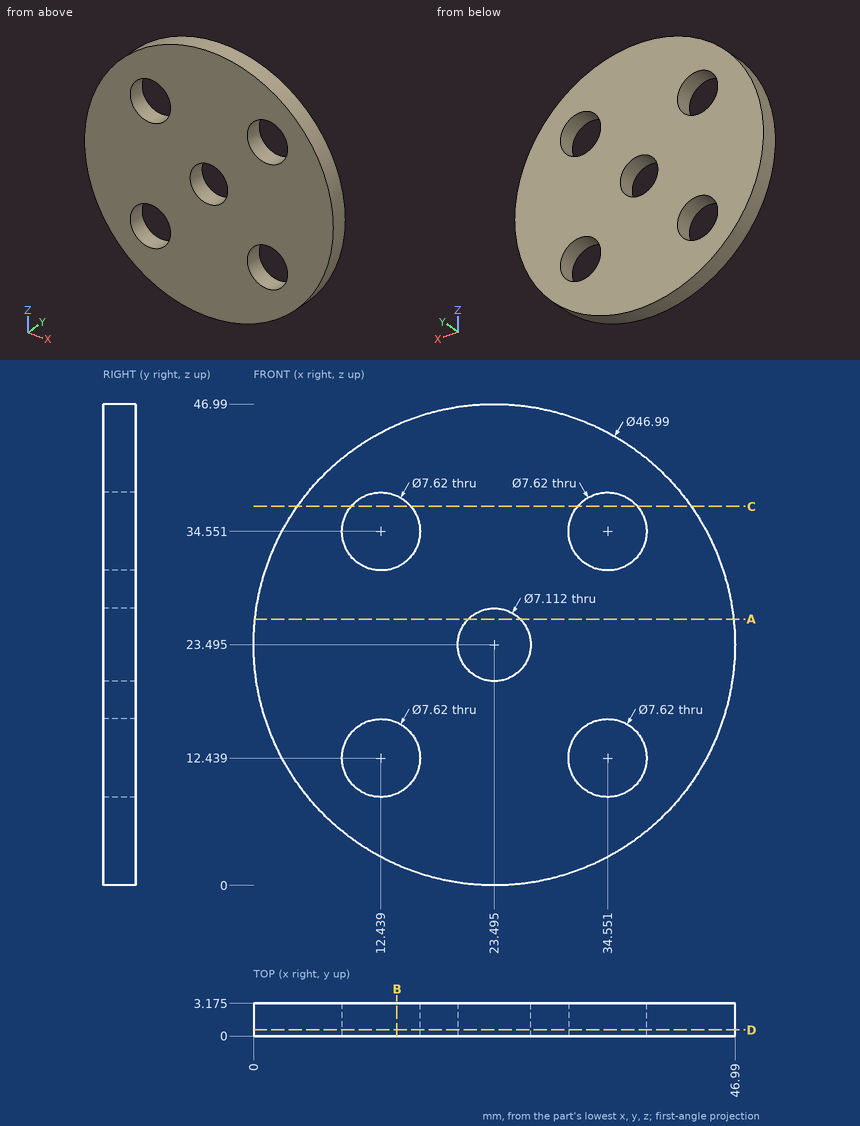
Study the drawing (mm; zero at the part's minimum x, y, z) and answer. Coordinates: 2 decimals unless noted, no trailing zeros. Write each loop counter-clockwise with the first axis right and the second up, starting at its lowest first coordinate (ties: lowest second). Pieces come first, ordered by that corner, then holes. Notation, with made-up numbers: (41.5, 45.5) - (71.5, 45.5) arc R17 cw to (71.5, 62.5) - close; hole circle Ø6 at (6, -38). An arc over 180 degrees is marked (long way). Return JSON: item names as keys, results as strings. Group by question number.
1. A cutting plane is placed at B-B, the plane x = 14. Determine the outline of the cut face in (y, z) (1 decimal), plus the area to 3 significant figures.
2. A cutting plane is placed at A-A, the plane z = 26. Determine the outline of the cut face in (x, y) (3 decimals), plus the area to 3 significant figures.
3. A cutting plane is placed at C-C, the plane z = 37. Determine the outline of the cut face in (x, y) (1 decimal).
4. Straight lines are drawn through the part: L1, parallel to X at y = 0.5, z = 10; L2, parallel to Z at x = 38, y = 2.4; L3, parallel to Z at x = 37, y = 1.55. For each, find the intervals that lie inside material, in ascending order.
5. A cutting plane is placed at D-D, the plane y = 0.6. Determine the outline of the cut face in (x, z) (3 decimals), plus the area to 3 significant figures.
6. Given pin 1 (10 mm diameter, centred on x = 12.44, z = 34.55, fed in from +Y) (3 decimals); pin 2 (1.5 mm diameter, centred on x = 22.5, y = 2.5, fed in from -Z); pin 3 (4.5 mm diameter, centred on x = 34.55, z = 34.55, fed in from +Y); pin 4 (1.5 mm diameter, centred on y = 0.5, z = 31, fed in from -X), each flat-ended and moving along its own axis, determine where each tip first touches the part or whether it passes through.
Ans:
{
 "1": {"outline": "(0, 2) - (3.2, 2) - (3.2, 9) - (0, 9) - close; (0, 15.9) - (3.2, 15.9) - (3.2, 31.1) - (0, 31.1) - close; (0, 38) - (3.2, 38) - (3.2, 45) - (0, 45) - close", "area": "92.3 mm²"},
 "2": {"outline": "(0.134, 0) - (20.971, 0) - (20.971, 3.175) - (0.134, 3.175) - close; (26.019, 0) - (46.856, 0) - (46.856, 3.175) - (26.019, 3.175) - close", "area": "132 mm²"},
 "3": {"outline": "(4.3, 0) - (9.5, 0) - (9.5, 3.2) - (4.3, 3.2) - close; (15.4, 0) - (31.6, 0) - (31.6, 3.2) - (15.4, 3.2) - close; (37.5, 0) - (42.7, 0) - (42.7, 3.2) - (37.5, 3.2) - close"},
 "4": {"L1": "4.26 to 9.51, 15.37 to 31.62, 37.48 to 42.73", "L2": "5.01 to 10.82, 14.06 to 32.93, 36.17 to 41.98", "L3": "4.27 to 9.52, 15.36 to 31.63, 37.47 to 42.72"},
 "5": {"outline": "circle Ø46.99 at (23.495, 23.495); hole circle Ø7.62 at (12.439, 12.439); hole circle Ø7.62 at (12.439, 34.551); hole circle Ø7.112 at (23.495, 23.495); hole circle Ø7.62 at (34.551, 12.439); hole circle Ø7.62 at (34.551, 34.551)", "area": "1,510 mm²"},
 "6": {"pin 1": "y = 3.175", "pin 2": "z = 0", "pin 3": "through", "pin 4": "x = 0.99"}
}
